```python
from build123d import *

# Parameters (mm, degrees)
BOSS_EXTRUDE1_START = 2
SKETCH1_R           = 5
SKETCH1_R_2         = 3
BOSS_EXTRUDE1_DEPTH = 2
BOSS_EXTRUDE2_START = 2
SKETCH2_R           = 3
BOSS_EXTRUDE2_DEPTH = 2
SKETCH3_W           = 75
SKETCH3_H           = 49
BOSS_EXTRUDE3_DEPTH = 2
SKETCH4_R           = 17.5
BOSS_EXTRUDE4_DEPTH = 8
SKETCH5_W           = 60
SKETCH5_H           = 60
BOSS_EXTRUDE5_DEPTH = 2


with BuildPart() as part:
    # Sketch1 → Boss-Extrude1 (new body)
    with BuildSketch(Plane.XY.offset(BOSS_EXTRUDE1_START)):
        with BuildLine():
            Line((50, 35), (-25, 35))
            Line((-25, 35), (-4.619219619, -1.91384694))
            ThreePointArc((-4.619219619, -1.91384694), (-0.975679739, 4.903881019), (5, 0))
            ThreePointArc((5, 0), (4.525827035, -2.125297543), (3.193244142, -3.847491631))
            Line((3.193244142, -3.847491631), (50, 35))
        make_face()
        Circle(SKETCH1_R)
        Circle(SKETCH1_R_2, mode=Mode.SUBTRACT)
    extrude(amount=BOSS_EXTRUDE1_DEPTH)



with BuildPart() as body_2:
    # Sketch2 → Boss-Extrude2 (new body)
    with BuildSketch(Plane(origin=(0, 0, -41), x_dir=(-1, 0, 0), z_dir=(0, 0, -1)).offset(BOSS_EXTRUDE2_START)):
        with BuildLine():
            ThreePointArc((-19.679195809, 9.835103065), (-4.101319052, 21.614328165), (14.708637674, 16.360194919))
            Line((14.708637674, 16.360194919), (25, 35))
            Line((25, 35), (-50, 35))
            Line((-50, 35), (-19.679195809, 9.835103065))
        make_face()
        with BuildLine():
            ThreePointArc((-3.193244142, -3.847491631), (1.201289708, -4.853545409), (4.619219619, -1.91384694))
            Line((4.619219619, -1.91384694), (14.708637674, 16.360194919))
            ThreePointArc((14.708637674, 16.360194919), (-4.101319052, 21.614328165), (-19.679195809, 9.835103065))
            Line((-19.679195809, 9.835103065), (-3.193244142, -3.847491631))
        make_face()
        Circle(SKETCH2_R, mode=Mode.SUBTRACT)
    extrude(amount=BOSS_EXTRUDE2_DEPTH)


with BuildPart() as part_1:
    add(part.part)

    add(body_2.part)  # Boss-Extrude3 merges body 2
    # Sketch3 → Boss-Extrude3 (add)
    with BuildSketch(Plane(origin=(0, 35, 0), x_dir=(1, 0, 0), z_dir=(0, 1, 0))):
        with Locations((12.5, 20.5)):
            Rectangle(SKETCH3_W, SKETCH3_H)
    extrude(amount=BOSS_EXTRUDE3_DEPTH)

    # Sketch4 → Boss-Extrude4 (add)
    with BuildSketch(Plane(origin=(0, 37, 0), x_dir=(1, 0, 0), z_dir=(0, 1, 0))):
        with Locations((32.5, 20.5)):
            Circle(SKETCH4_R)
    extrude(amount=BOSS_EXTRUDE4_DEPTH)

    # Sketch5 → Boss-Extrude5 (add)
    with BuildSketch(Plane(origin=(0, 45, 0), x_dir=(1, 0, 0), z_dir=(0, 1, 0))):
        with Locations((32.5, 20.5)):
            Rectangle(SKETCH5_W, SKETCH5_H)
        with BuildLine():
            Line((9.5, 47.742640687), (13.742640687, 43.5))
            ThreePointArc((13.742640687, 43.5), (13.742640687, 39.257359313), (9.5, 39.257359313))
            Line((9.5, 39.257359313), (5.257359313, 43.5))
            ThreePointArc((5.257359313, 43.5), (5.257359313, 47.742640687), (9.5, 47.742640687))
        make_face(mode=Mode.SUBTRACT)
        with BuildLine():
            Line((59.742640687, 43.5), (55.5, 39.257359313))
            ThreePointArc((55.5, 39.257359313), (51.257359313, 39.257359313), (51.257359313, 43.5))
            Line((51.257359313, 43.5), (55.5, 47.742640687))
            ThreePointArc((55.5, 47.742640687), (59.742640687, 47.742640687), (59.742640687, 43.5))
        make_face(mode=Mode.SUBTRACT)
        with BuildLine():
            Line((55.5, -6.742640687), (51.257359313, -2.5))
            ThreePointArc((51.257359313, -2.5), (51.257359313, 1.742640687), (55.5, 1.742640687))
            Line((55.5, 1.742640687), (59.742640687, -2.5))
            ThreePointArc((59.742640687, -2.5), (59.742640687, -6.742640687), (55.5, -6.742640687))
        make_face(mode=Mode.SUBTRACT)
        with BuildLine():
            Line((5.257359313, -2.5), (9.5, 1.742640687))
            ThreePointArc((9.5, 1.742640687), (13.742640687, 1.742640687), (13.742640687, -2.5))
            Line((13.742640687, -2.5), (9.5, -6.742640687))
            ThreePointArc((9.5, -6.742640687), (5.257359313, -6.742640687), (5.257359313, -2.5))
        make_face(mode=Mode.SUBTRACT)
    extrude(amount=BOSS_EXTRUDE5_DEPTH)


solid = part_1.part
```
Work out the finished part from the listing and answer in its coordinate system (mm). A direction names the side the tool comes from. Coordinates: 2 decimals unless noted, no trailing zeros. Write each loop counter-clockwise with the first axis right and the second up, starting at its lowest first coordinate (ties: lowest second). Pieces come first, ordered by that corner, then holes.
Q1. A cutting plane is placed at D-D, the plane x = 25.5. Give the vertices of the cut face in (y, z).
Q2. A cutting plane is placed at B-B, the plane x = 0. Give the vertices of the cut face in (y, z).
Q3. A cutting plane is placed at A-A, the plane z = -34.5. Give the vertices of the cut face in (x, y), then the cut area to 3 significant figures.
Q4. A cutting plane is placed at C-C, the plane y = 29.5. Give the vertices of the cut face in (x, z), then the cut area to 3 significant figures.
Q5. Each of these flat-tipped pins is pushed along its axis until it touches: pin 1 Ø1 at (x, y) = (25.5, 34.5) entering from +Z; pin 2 Ø8 at (y, z) = (6.5, 0.5) entering from -X; pin 3 Ø5 at (x, z) = (27, -10) entering from -Y. Where does it stop, or does it pass through?
Q6. Find the intervals of material crossed by line 1 (Z direction, x = 34, y = 32); line 2 (Y direction, x = 0, z = 3); line 3 (Y direction, x = -15, z = 1), in increasing order.
Q7. Which of the six approach directions +Z, -Z, +X, -X, +Y, -Y give full straight-line access (tool end or side, diameter ignored) to faces 5 (the face through (5.211, 45.986, -47.695)), 6 (the face through (4, 20, 2)), 7 (the face through (19, 45, -34))?
Q8. Determine the mould class of faces 1 (the face through (32, 46, 9.5)), 2 (the face through (50, 36, -20)), 3 (the face through (53.35, 45.99, -45.59)), 4 (the face through (13.695, 45.986, -1.789)) for opening direction X: released by +X, released by -X, zero draft, split by the parting line, or undercut.
Findings below:
1. outline: (14.67, -45) - (37, -45) - (37, -36.54) - (45, -36.54) - (45, -50.5) - (47, -50.5) - (47, 9.5) - (45, 9.5) - (45, -4.46) - (37, -4.46) - (37, 4) - (14.67, 4) - (14.67, 2) - (35, 2) - (35, -43) - (14.67, -43) - close
2. outline: (-5, -45) - (-3, -45) - (-3, -43) - (-5, -43) - close; (-5, 2) - (-3, 2) - (-3, 4) - (-5, 4) - close; (3, -45) - (37, -45) - (37, 4) - (3, 4) - (3, 2) - (35, 2) - (35, -43) - (3, -43) - close
3. outline: (-25, 35) - (50, 35) - (50, 37) - (43, 37) - (43, 45) - (62.5, 45) - (62.5, 47) - (2.5, 47) - (2.5, 45) - (22, 45) - (22, 37) - (-25, 37) - close
3. area: 438 mm2
4. outline: (-21.96, -45) - (43.37, -45) - (43.37, -43) - (-21.96, -43) - close; (-21.96, 2) - (43.37, 2) - (43.37, 4) - (-21.96, 4) - close
4. area: 261 mm2
5. pin 1: stops at z = 4
5. pin 2: stops at x = -11.31
5. pin 3: stops at y = 35
6. line 1: z = -45 to -43, 2 to 4
6. line 2: y = -5 to -3, 3 to 37
6. line 3: y = 35 to 37
7. face 5: +Y
7. face 6: +X, -X, -Y
7. face 7: none
8. face 1: zero draft
8. face 2: released by +X
8. face 3: undercut
8. face 4: undercut
